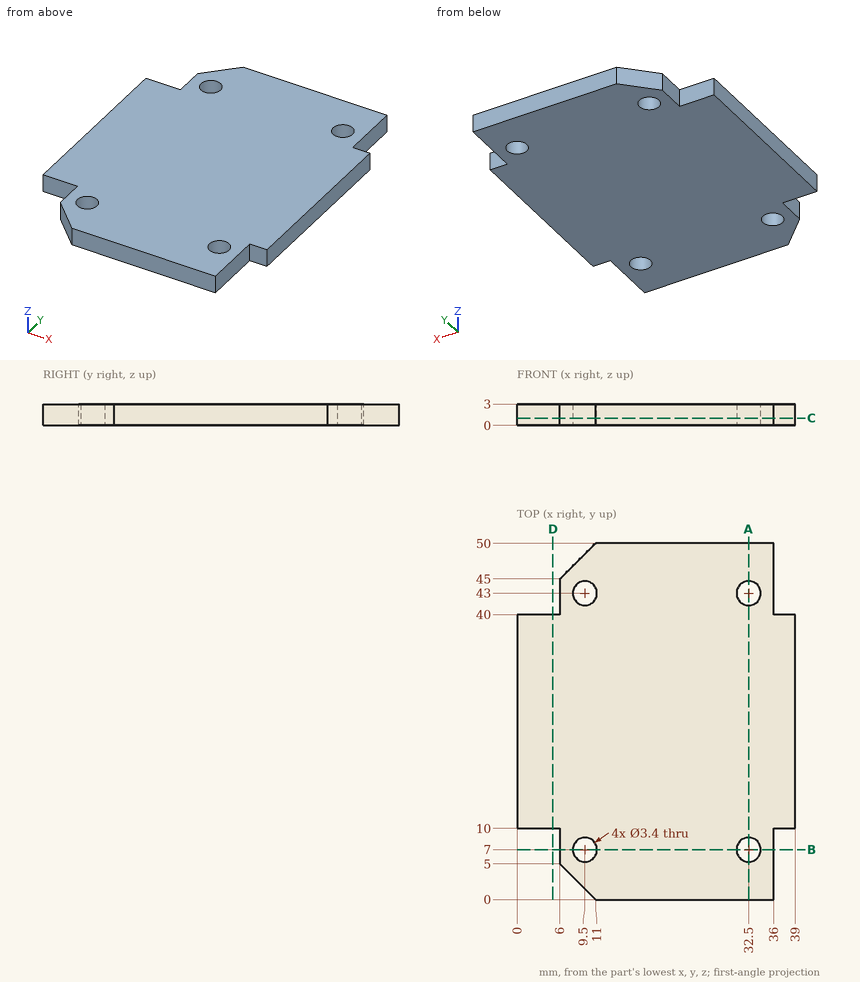
Job drawing, mm, ordinate dimensions from the low corner. One solid piece. Give positions to 0.01 mm unless a question says otherwise; leave off trailing zeros. Write each loop counter-clockwise with the first axis right and the second up, starting at its lowest first coordinate (ties: lowest second). Pieces come first, ordered by that corner, then holes. Notation, with made-up numbers: M -4,4 L 22,4 A23 cw 22,39 Z; hole C -32,48 d5. An arc over 180 degrees is marked long. One line per item, written item: value. Start each with the question number.
Q1. Saw through at B-B, the plane y = 7. Write the cut outline in (x, z).
Q2. Drop flat-ended pins along their axis: pin 1 Ø1.5 at (y, z) = (42.5, 1) entering from -X; pin 2 Ø1.5 at (x, z) = (37.5, 1.5) entering from +Y; pin 3 Ø0.9 at (y, z) = (44.5, 1) entering from +X. Give the stop position or say it passes through.
Q3. Saw through at A-A, the plane x = 32.5. Write the cut outline in (y, z), plus the area to 3 significant figures.
Q4. Probe probe 1 along Y at (x, z) = (32.5, 1.9); probe 2 along Y at (x, z) = (9.5, 1.55); probe 3 along Y at (x, z) = (5, 0.5). List the from-to ranges inside material, lowest first. Write a range as [from, to].
Q5. Saw through at C-C, the plane z = 1. Write the cut outline in (x, y), plus the area to 3 significant figures.
Q6. Saw through at D-D, the plane x = 5. Write the cut outline in (y, z).
Output values:
1. outline: M 6,0 L 7.8,0 L 7.8,3 L 6,3 Z; M 11.2,0 L 30.8,0 L 30.8,3 L 11.2,3 Z; M 34.2,0 L 36,0 L 36,3 L 34.2,3 Z
2. pin 1: stops at x = 6
2. pin 2: stops at y = 40
2. pin 3: stops at x = 36
3. outline: M 0,0 L 5.3,0 L 5.3,3 L 0,3 Z; M 8.7,0 L 41.3,0 L 41.3,3 L 8.7,3 Z; M 44.7,0 L 50,0 L 50,3 L 44.7,3 Z
3. area: 130 mm²
4. probe 1: y = [0, 5.3], [8.7, 41.3], [44.7, 50]
4. probe 2: y = [1.5, 5.3], [8.7, 41.3], [44.7, 48.5]
4. probe 3: y = [10, 40]
5. outline: M 0,10 L 6,10 L 6,5 L 11,0 L 36,0 L 36,10 L 39,10 L 39,40 L 36,40 L 36,50 L 11,50 L 6,45 L 6,40 L 0,40 Z; hole C 9.5,7 d3.4; hole C 9.5,43 d3.4; hole C 32.5,7 d3.4; hole C 32.5,43 d3.4
5. area: 1,710 mm²
6. outline: M 10,0 L 40,0 L 40,3 L 10,3 Z
